Design review of the part built by this model. Coordinates are the model's own, in mm. A direction names the side the tool comes from. Give positions to 0.01 mm unless a question says otherwise; leave off trailing zeros. Loops run counter-clockwise (first coordinate to the right, second up) from the corner with the lowest first, then second, coordinate; pieces in that order, holes last. Notation, with made-up numbers: (79.25, 73.5) - (100.25, 73.5) arc R30 cw to (100.25, 106.5) - close; hole circle Ø8 at (75.25, 46.25). An arc over 180 degrees is marked (long way). Write each question's results on one line, items separated by ' | '.
from build123d import *

# Parameters (mm, degrees)
F0_W     = 35
F0_H     = 30
F0_R     = 1.3
F0_R_2   = 12
F0_R_3   = 11
F1_DEPTH = 3
F3_DEPTH = 7.75
F4_R     = 7.74999
F5_DEPTH = 5


# Not quite as in the source:
# - a fillet or chamfer is up to 0.001 mm smaller than in the source, because OpenCascade refuses the exact size


with BuildPart() as f1:
    # F0 (on Front) → F1 (new body)
    with BuildSketch(Plane.XZ):
        Rectangle(F0_W, F0_H)
        with Locations((-12.5, -12.5)):
            Circle(F0_R, mode=Mode.SUBTRACT)
        with Locations((12.5, -12.5)):
            Circle(F0_R, mode=Mode.SUBTRACT)
        with Locations((-12.5, 12.5)):
            Circle(F0_R, mode=Mode.SUBTRACT)
        Circle(F0_R_2, mode=Mode.SUBTRACT)
        with Locations((12.5, 12.5)):
            Circle(F0_R, mode=Mode.SUBTRACT)
        Circle(F0_R_2)
        Circle(F0_R_3, mode=Mode.SUBTRACT)
        Circle(F0_R_3)
    extrude(amount=F1_DEPTH)

    # F2 (on Right) → F3 (cut, symmetric)
    with BuildSketch(Plane.YZ):
        Polygon((24.7599773954, -16.2912994583), (30.0612896169, -1.7260638362), (-14.6986877785, 14.5652356222), (-20, 0), align=None)
    extrude(amount=F3_DEPTH, both=True, mode=Mode.SUBTRACT)

    # F4 (radius 7.75 in the source; OpenCascade refuses exactly that, so slightly less here)
    f4_edges = [f1.edges().sort_by_distance(p)[0] for p in [
        (7.75, -1.5, 9.761306),
        (-7.75, -1.5, 9.761306),
        (-7.75, -1.5, -6.733449),
        (7.75, -1.5, -6.733449),
    ]]
    fillet(f4_edges, radius=F4_R)

    # F0 (on Front) → F5 (join)
    with BuildSketch(Plane.XZ):
        Circle(F0_R_2)
        Circle(F0_R_3, mode=Mode.SUBTRACT)
    extrude(amount=F5_DEPTH)


solid = f1.part
(1) Take a section at B-B on x = 12.5. Give the boundary of the cut face in (y, z).
Answers below:
outline: (-3, -15) - (0, -15) - (0, -13.8) - (-3, -13.8) - close; (-3, -11.2) - (0, -11.2) - (0, 11.2) - (-3, 11.2) - close; (-3, 13.8) - (0, 13.8) - (0, 15) - (-3, 15) - close
(2) Take a section at D-D on z = -10.5. Give the boundary of the cut face in (x, y).
Answers below:
outline: (-17.5, -3) - (-5.81, -3) - (-5.81, -5) - (-3.28, -5) - (-3.28, -3) - (3.28, -3) - (3.28, -5) - (5.81, -5) - (5.81, -3) - (17.5, -3) - (17.5, 0) - (-17.5, 0) - close
(3) Take a section at A-A on z = 12.5. Give the boundary of the cut face in (x, y).
Answers below:
outline: (-17.5, -3) - (-13.8, -3) - (-13.8, 0) - (-17.5, 0) - close; (-11.2, -3) - (11.2, -3) - (11.2, 0) - (-11.2, 0) - close; (13.8, -3) - (17.5, -3) - (17.5, 0) - (13.8, 0) - close
(4) Draft analysis for pull direction X (two halves, no side actions). For faces 1 (the cylindrical face through (-11.99, -3.99, 0.53)), 2 (the flat face through (0, -1, 15)), 3 (the cylindrical face through (-12.67, -1.48, 13.79)), state which applies: pulls with the +X half, pulls with the -X half, needs draft (parallel to the pull), parting line crosses it, or undercut.
Answers below:
face 1: parting line crosses it | face 2: needs draft | face 3: undercut
(5) Tool access review of faces 4 (the flat face through (0, -3, -7)), 5 (the flat face through (17.5, -1, 0)): name each direction out of +Z, -Z, +X, -X, +Y, -Y from which nothing blocks a thin tool from reaching the whole face with its end or side.
Answers below:
face 4: -Y | face 5: +Z, -Z, +X, +Y, -Y
(6) Insertion check: P1, Ø3, axis at x = 12.5, z = -12.5, coming from the -Y side. The pin has a flat end and moves straight along its axis. Give the tip position at first contact, or say it passes through.
Answers below:
P1: y = -3
(7) Wall thickness on line 1 along X through (y, z) = (-3.6, 0); line 2 along X through (y, z) = (-1.35, 1.5); line 3 along Z through (x, y) = (-12.5, -0.65): over which ranges is each line inside the solid? List them lowest first. Write a range as from..to.
Answers below:
line 1: -12..-11, 11..12 | line 2: -17.5..-7.75, 7.75..17.5 | line 3: -15..-13.8, -11.2..11.2, 13.8..15
(8) Take a section at C-C on y = -3.8. Give the boundary of the cut face in (x, z).
Answers below:
outline: circle Ø24 at (0, 0); hole circle Ø22 at (0, 0)
